Source: CAD feature listing. Evaluate the final solid. Frame: model axes, mm. Coordinates: 2 decimals unless noted, no trailing zeros. Order: outer loops, then holes, each group sorted by start corner. A loop starts at its lowest first (then second) coordinate and runs counter-clockwise, first axis right, second up. Notation, with made-up numbers: (16.25, -3) - (73.25, -3) arc R11 ccw to (73.25, 18) - close; hole circle Ø6 at (74, 21.25). An arc over 180 degrees is marked (long way). One line per question, with ' | ' between items. Start each with the question number.
(1) Section B-B (y = 0.9). Return the cut outline in (x, z).
(2) Line query: line 1 along X through (y, z) = (1.35, -40.5); line 2 along X through (y, z) = (0.3, -43); line 3 along Z through (x, y) = (-45.5, 0.6). Output: solid intervals per line, ascending.
(3) Section A-A (x = -56). Return the cut outline in (y, z).
(4) Draft query along X for faces 1 (the cylindrical face through (-50.765, 2.128, -41.935)), 2 (the flat face through (-60.755, 1, -42)), 3 (the flat face through (-51, 1, -52.075)). Return one class per face: +X half, -X half, draft (parallel to the pull), parting line (faces both ways), or undercut.
from build123d import *

# Parameters (mm, degrees)
SKETCH1_W           = 20
SKETCH1_H           = 20
BOSS_EXTRUDE1_DEPTH = 2.5
SKETCH2_R           = 0.6223
CUT_EXTRUDE1_DEPTH  = 21
SKETCH3_R           = 2
CUT_EXTRUDE2_DEPTH  = 3.5


with BuildPart() as part:
    # Sketch1 → Boss-Extrude1 (new body)
    with BuildSketch(Plane(origin=(0, 0, 0), x_dir=(1, 0, 0), z_dir=(0, 1, 0))):
        with Locations((-50.754716981, 42.075471698)):
            Rectangle(SKETCH1_W, SKETCH1_H)
    extrude(amount=BOSS_EXTRUDE1_DEPTH)

    # Sketch2 → Cut-Extrude1 (cut, through all)
    with BuildSketch(Plane.XY.offset(-32.075471698)):
        with Locations((-50.754716981, 2.75)):
            Circle(SKETCH2_R)
    extrude(amount=-CUT_EXTRUDE1_DEPTH, mode=Mode.SUBTRACT)

    # Sketch3 → Cut-Extrude2 (cut, through all)
    with BuildSketch(Plane(origin=(0, 2.5, 0), x_dir=(1, 0, 0), z_dir=(0, 1, 0))):
        with Locations((-55.754716981, 42.075471698)):
            Circle(SKETCH3_R)
        with Locations((-45.754716981, 42.075471698)):
            Circle(SKETCH3_R)
    extrude(amount=-CUT_EXTRUDE2_DEPTH, mode=Mode.SUBTRACT)


solid = part.part
Response values:
1) outline: (-60.75, -52.08) - (-40.75, -52.08) - (-40.75, -32.08) - (-60.75, -32.08) - close; hole circle Ø4 at (-55.75, -42.08); hole circle Ø4 at (-45.75, -42.08)
2) line 1: x = -60.75 to -56.99, -54.52 to -46.99, -44.52 to -40.75 | line 2: x = -60.75 to -57.53, -53.98 to -47.53, -43.98 to -40.75 | line 3: z = -52.08 to -44.06, -40.09 to -32.08
3) outline: (0, -52.08) - (2.5, -52.08) - (2.5, -44.06) - (0, -44.06) - close; (0, -40.09) - (2.5, -40.09) - (2.5, -32.08) - (0, -32.08) - close
4) face 1: undercut | face 2: -X half | face 3: draft
